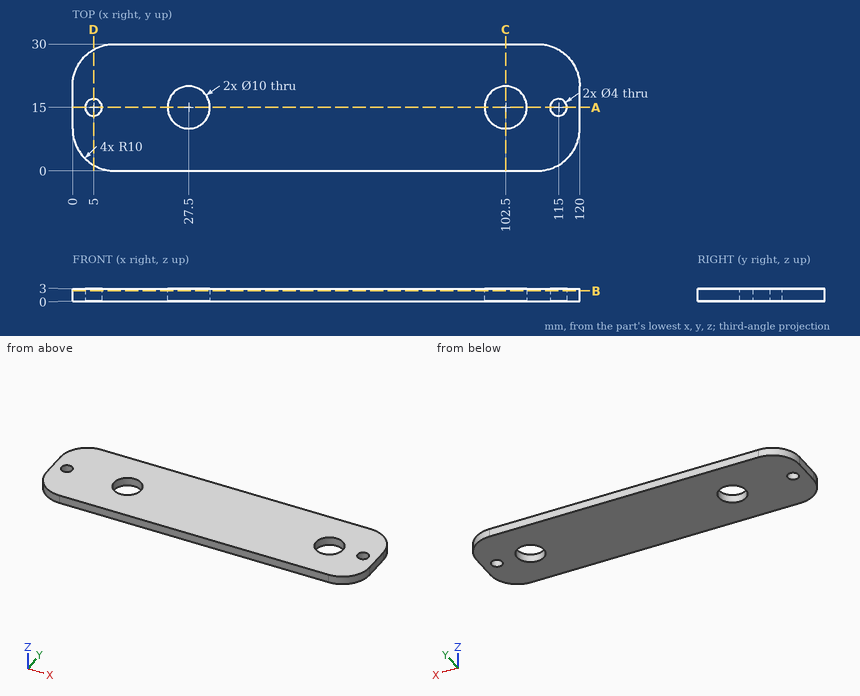
Check sheet for the drawn part. Datum: minimum x, y, z corner. Units: mm. Round coordinates to 2 decimals unless told otherwise and drop trailing zeros. Order: outer loops, then holes, each group sorted by start corner. A loop starts at its lowest first (then second) coordinate and runs counter-clockwise, first axis right, second up. Notation, with made-up numbers: (-38.5, 5.5) -> (-7.5, 5.5) arc R8 ccw to (-7.5, 16.5) -> close; hole circle Ø1 at (-29, 89.25). An arc over 180 degrees is marked (long way). Return JSON: item names as keys, results as strings. Group by question number.
Q1. Section check B-B, the plane z = 2.5. Record the boundary of the cut face in (x, y), plus the area to 3 significant figures.
Q2. Section check C-C, the plane x = 102.5. Record the boundary of the cut face in (y, z), plus the area to 3 significant figures.
Q3. Section check D-D, the plane x = 5. Record the boundary of the cut face in (y, z), plus the area to 3 significant figures.
Q4. Material ranges on probe 1 along X at (y, z) = (15.5, 0.2); probe 2 along X at (y, z) = (11.75, 0.15); probe 3 along Y at (x, z) = (5, 1.25), recorded low to high. Write a range as from..to.
Q5. Section check A-A, the plane y = 15. Record the boundary of the cut face in (x, z), plus the area to 3 significant figures.
Q6. Gauge pin test, flat end, axial feed: pin 1 (1 mm diameter, centred on x = 101.5, y = 10, fed in from -Z). Record the tip position at first contact, or that the pin passes through.
Numbers:
{
 "1": {"outline": "(0, 10) arc R10 ccw to (10, 0) -> (110, 0) arc R10 ccw to (120, 10) -> (120, 20) arc R10 ccw to (110, 30) -> (10, 30) arc R10 ccw to (0, 20) -> close; hole circle Ø4 at (5, 15); hole circle Ø10 at (27.5, 15); hole circle Ø10 at (102.5, 15); hole circle Ø4 at (115, 15)", "area": "3,330 mm^2"},
 "2": {"outline": "(0, 0) -> (10, 0) -> (10, 3) -> (0, 3) -> close; (20, 0) -> (30, 0) -> (30, 3) -> (20, 3) -> close", "area": "60.0 mm^2"},
 "3": {"outline": "(1.34, 0) -> (13, 0) -> (13, 3) -> (1.34, 3) -> close; (17, 0) -> (28.66, 0) -> (28.66, 3) -> (17, 3) -> close", "area": "70.0 mm^2"},
 "4": {"probe 1": "0..3.06, 6.94..22.53, 32.47..97.53, 107.47..113.06, 116.94..120", "probe 2": "0..23.7, 31.3..98.7, 106.3..120", "probe 3": "1.34..13, 17..28.66"},
 "5": {"outline": "(0, 0) -> (3, 0) -> (3, 3) -> (0, 3) -> close; (7, 0) -> (22.5, 0) -> (22.5, 3) -> (7, 3) -> close; (32.5, 0) -> (97.5, 0) -> (97.5, 3) -> (32.5, 3) -> close; (107.5, 0) -> (113, 0) -> (113, 3) -> (107.5, 3) -> close; (117, 0) -> (120, 0) -> (120, 3) -> (117, 3) -> close", "area": "276 mm^2"},
 "6": {"pin 1": "z = 0"}
}
